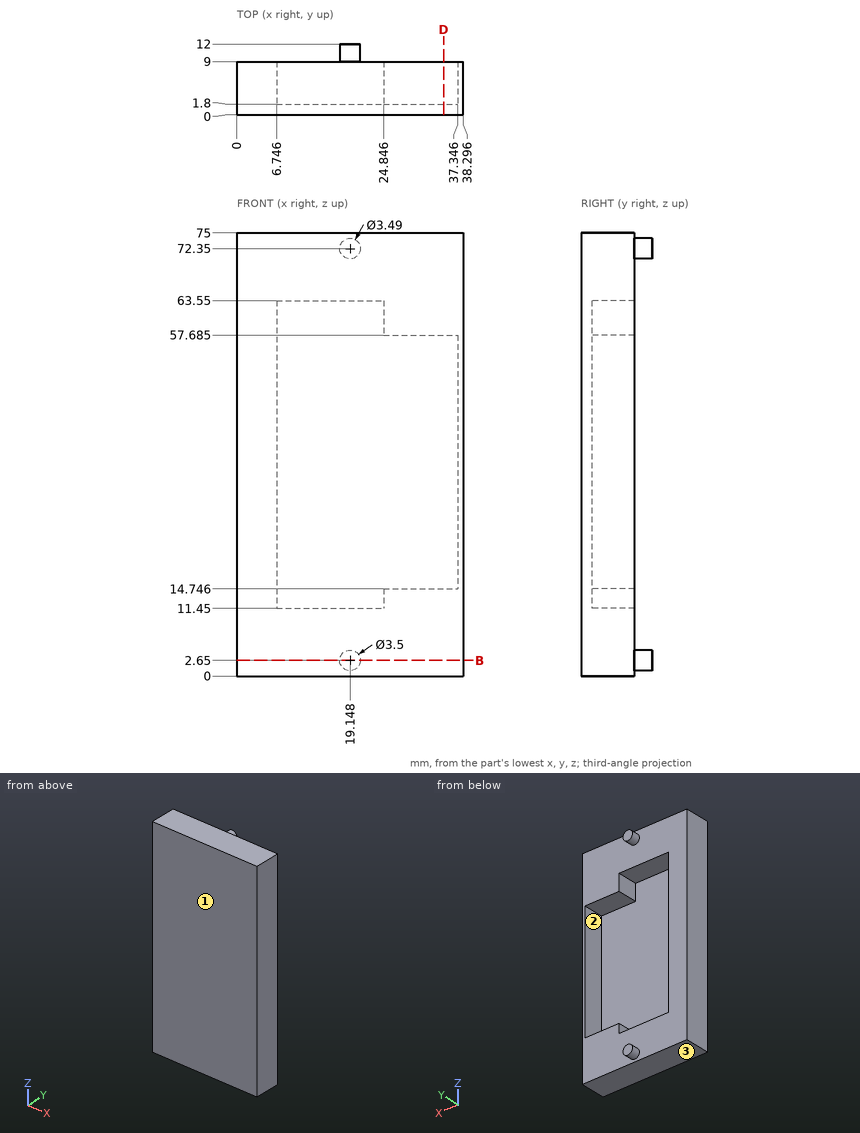
Answer from the drawing. Dimensions are ordinates in mm from the lowest x, y and z of the part. Give positions to 0.01 mm unless a question says otherwise; leave off trailing zeros. Loops run counter-clockwise (first coordinate to the right, second up) from the corner with the lowest first, then second, coordinate; pieces in that order, holes last. Notation, with made-up numbers: (-33, -14) -> (25, -14) arc R16 cw to (25, -10) -> close; hole circle Ø6 at (7, 17.25). An arc over 180 degrees is marked (long way). Answer as CSV lines item,"result".
Item 1: Each of these flat-tipped pins is pushed along its axis until it touches: pin 1 (11.5 mm diameter, centred on x = 18, z = 39, fed in from +Y); pin 2 (3 mm diameter, centred on x = 24, z = 15, fed in from +Y). Where does it stop, or does it pass through?
Returned:
pin 1,"stops at y = 1.8"
pin 2,"stops at y = 9"
Item 2: Determine the mould class of the marked faces 1, 2 and 3 for opening direction Z: +Z half, -Z half, draft (parallel to the pull), parting line (faces both ways), or undercut.
Returned:
face 1,"draft"
face 2,"undercut"
face 3,"-Z half"
Item 3: Consider line 1 (Z direction, x = 32, y = 5.5) (1 decimal); line 2 (Z direction, x = 10, y = 2.25); line 3 (X direction, y = 6, z = 21.5) (1 decimal). Determine where each line is inside the solid, lowest interval first. Write a range as [from, to].
Returned:
line 1,"z = [0, 14.7], [57.7, 75]"
line 2,"z = [0, 11.45], [63.55, 75]"
line 3,"x = [0, 6.7], [37.3, 38.3]"
Item 4: Find section B-B on z = 2.65. Give the vertices of the cut face in (x, y) (1 decimal), plus the area to 3 significant figures.
Returned:
outline,"(0, 0) -> (38.3, 0) -> (38.3, 9) -> (20.9, 9) -> (20.9, 12) -> (17.4, 12) -> (17.4, 9) -> (0, 9) -> close"
area,"355 mm²"
Item 5: Find section D-D on x = 35. Give the vertices of the cut face in (y, z) (1 decimal), plus the area to 3 significant figures.
Returned:
outline,"(0, 0) -> (9, 0) -> (9, 14.7) -> (1.8, 14.7) -> (1.8, 57.7) -> (9, 57.7) -> (9, 75) -> (0, 75) -> close"
area,"366 mm²"
